Here's how the part is built. I have some questions about the finished solid (model axes, mm). A direction names the side the tool comes from. Round coordinates to 2 decimals unless told otherwise and drop trailing zeros. Order: outer loops, then holes, each group sorted by start corner. A loop starts at its lowest first (then second) coordinate and runs counter-clockwise, first axis right, second up. Notation, with made-up numbers: (57, -25.5) -> (98, -25.5) arc R12 ccw to (98, -12.5) -> close; hole circle Ø3 at (-39.5, -21.75). An arc over 180 degrees is marked (long way). Use a Markdown table: item, result. Add a question column.
(1) I want a section at C-C, the plane x = 0. Please give me the cut outline in (y, z), then the cut area to 3 significant figures.
(2) I want a section at D-D, the plane x = 76.5. Please give me the cut outline in (y, z).
(3) If I drill on probe 1 along X at (y, z) = (-3.4, 22); probe 2 along X at (y, z) = (-4.6, -119.5); probe 3 along X at (y, z) = (-3.2, 12.5), over which ranges is the centre line in solid material (lowest first)?
(4) On a 3-axis mill with a long thin cutter (end or side, diameter ignored), from which of +Z, -Z, +X, -X, +Y, -Y can I reach the whole of each face in a straight line? I mean faces 5 (the face through (-46.428, -2.465, 47.716)), 6 (the face through (-19.524, -2.535, 4.336)). Say none if no direction works.
(5) Thinking about a two-plate mould opening in Z: for faces 1 (the face through (-100.65, -2.46, -18.11)), 2 (the face through (-4, -5, 22)), 3 (the face through (55.11, -2.46, -30.99)), 4 (the face through (51.164, -2.465, 54.543)), which applies, pulls with the +Z half, pulls with the -Z half, needs draft (parallel to the pull), parting line crosses it, or undercut?
(6) I'm going to push flat-ended pins straight in: P1, Ø1, axis at y = -1.5, z = -71.5, coming from the -X side; P2, Ø3.5, axis at x = -151.95, z = 21.9, coming from the -Y side; P3, Ø1, axis at y = -4, z = 9, coming from the -X side; P4, Ø1.5, axis at y = -2, z = -127, coming from the -X side. Where does each tip first touch, or does it pass through?
(7) I want a section at B-B, the plane y = -3.2. Give the number of separate pieces and of enclosed holes in the cut face, then the cut area to 3 significant figures.
(8) I want a section at A-A, the plane z = -30. Please give me the cut outline in (x, y), then the cut area to 3 significant figures.
from build123d import *

# Parameters (mm, degrees)
EXTRUDE_1_DEPTH        = 5
SKETCH_3_R             = 20
CUT_EXTRUDE_1_DEPTH    = 221.897762361
HOLE_WIZARD_M6_1_D     = 6.6
HOLE_WIZARD_M4_2_D     = 4.5
HOLE_WIZARD_M4_2_DEPTH = 10
HOLE_WIZARD_M4_2_TIP   = 1.351936393


with BuildPart() as part:
    # 스케치2 → 보스-돌출1 (new body)
    with BuildSketch(Plane(origin=(0, 0, 0), x_dir=(1, 0, 0), z_dir=(0, 1, 0))):
        with BuildLine():
            Line((66.01, 8.662039246), (66.01, 149.538220784))
            Line((66.01, 149.538220784), (28.01, 149.538220784))
            Line((28.01, 149.538220784), (28.01, 86.204565384))
            ThreePointArc((28.01, 86.204565384), (21.482045359, 71.422684791), (6.159600614, 66.290348801))
            ThreePointArc((6.159600614, 66.290348801), (-18.444176134, 63.970019467), (-40.506546036, 52.835317281))
            Line((-40.506546036, 52.835317281), (-162.508898036, -17.602773488))
            Line((-162.508898036, -17.602773488), (-143.508898036, -50.511738832))
            Line((-143.508898036, -50.511738832), (-88.660343545, -18.844911132))
            ThreePointArc((-88.660343545, -18.844911132), (-72.594882115, -17.10734539), (-60.488926395, -27.810803791))
            ThreePointArc((-60.488926395, -27.810803791), (-46.177573873, -47.958134817), (-25.503453964, -61.497356527))
            Line((-25.503453964, -61.497356527), (96.498898036, -131.935447296))
            Line((96.498898036, -131.935447296), (115.498898036, -99.026481952))
            Line((115.498898036, -99.026481952), (60.650343545, -67.359654252))
            ThreePointArc((60.650343545, -67.359654252), (51.112836757, -54.315339401), (54.32932578, -38.47954501))
            ThreePointArc((54.32932578, -38.47954501), (64.621750006, -16.01188465), (66.01, 8.662039246))
        make_face()
    extrude(amount=-EXTRUDE_1_DEPTH)

    # 스케치3 → 컷-돌출1 (cut, through all)
    with BuildSketch(Plane(origin=(0, -5, 0), x_dir=(-1, 0, 0), z_dir=(0, -1, 0))):
        with Locations(Location((0, 0, 0), (0, 0, 90))):
            Circle(SKETCH_3_R)
    extrude(amount=-CUT_EXTRUDE_1_DEPTH, mode=Mode.SUBTRACT)

    # M6 여유 구멍1 (through all)
    with Locations(Plane(origin=(0, -5, 0), x_dir=(-1, 0, 0), z_dir=(0, -1, 0))):
        with Locations((30.310889132, 17.5), (0, -60), (0, -35), (-51.961524227, 30), (-30.310889132, 17.5), (51.961524227, 30)):
            Hole(HOLE_WIZARD_M6_1_D / 2)

    # M4 여유 구멍2
    with Locations(Plane(origin=(0, 0, 0), x_dir=(1, 0, 0), z_dir=(0, 1, 0))):
        with Locations((57.01, 142.538220784), (37.01, 142.538220784), (37.01, 70.038220784), (57.01, 70.038220784), (94.936720209, -120.641218662), (104.936720209, -103.320710586), (42.149878435, -67.070710586), (32.149878435, -84.391218662), (-151.946720209, -21.897002122), (-141.946720209, -39.217510198), (-79.159878435, -2.967510198), (-89.159878435, 14.352997878)):
            Hole(HOLE_WIZARD_M4_2_D / 2, depth=HOLE_WIZARD_M4_2_DEPTH)
            with Locations((0, 0, -(HOLE_WIZARD_M4_2_DEPTH + HOLE_WIZARD_M4_2_TIP / 2))):  # 118° drill point
                Cone(0, HOLE_WIZARD_M4_2_D / 2, HOLE_WIZARD_M4_2_TIP, mode=Mode.SUBTRACT)


solid = part.part
Taken from the geometry:
| question | item | result |
|---|---|---|
| 1 | outline | (-5, -66.58) -> (0, -66.58) -> (0, -20) -> (-5, -20) -> close; (-5, 20) -> (0, 20) -> (0, 31.7) -> (-5, 31.7) -> close; (-5, 38.3) -> (0, 38.3) -> (0, 56.7) -> (-5, 56.7) -> close; (-5, 63.3) -> (0, 63.3) -> (0, 76.22) -> (-5, 76.22) -> close |
| 1 | area | 448 mm2 |
| 2 | outline | (-5, 76.51) -> (0, 76.51) -> (0, 120.39) -> (-5, 120.39) -> close |
| 3 | probe 1 | x = -159.97 to -154.19, -149.7 to -94.13, -64.54 to 62.84 |
| 3 | probe 2 | x = 28.01 to 66.01 |
| 3 | probe 3 | x = -153.67 to -15.61, 15.61 to 65.39 |
| 4 | face 5 | +Z, +Y, -Y |
| 4 | face 6 | +Y, -Y |
| 5 | face 1 | pulls with the -Z half |
| 5 | face 2 | needs draft |
| 5 | face 3 | undercut |
| 5 | face 4 | undercut |
| 6 | P1 | stops at x = 21 |
| 6 | P2 | passes through |
| 6 | P3 | stops at x = -148.47 |
| 6 | P4 | stops at x = 28.01 |
| 7 | separate pieces | 1 |
| 7 | enclosed holes | 19 |
| 7 | area | 24,700 mm2 |
| 8 | outline | (-80.06, -5) -> (-55.26, -5) -> (-55.26, 0) -> (-80.06, 0) -> close; (-48.66, -5) -> (48.66, -5) -> (48.66, 0) -> (-48.66, 0) -> close; (55.26, -5) -> (66.01, -5) -> (66.01, 0) -> (55.26, 0) -> close |
| 8 | area | 664 mm2 |
